Verification items for the finished model (mm, model axes). A direction names the side the tool comes from. Give positions to 0.01 mm unless a question says otherwise; leave off trailing zeros. Order: outer loops, then holes, each group sorted by start corner. A loop starts at its lowest first (then second) coordinate and runs counter-clockwise, first axis right, second up. Notation, with made-up numbers: (84, -37) - (121, -37) arc R11 ccw to (121, -22) - close; hole circle Ø8 at (65, -15.75). An arc over 180 degrees is marked (long way). Answer as a JSON object with one key per item and string values. Group by question number.
(1) Section check C-C (y = 82.5). Record the boundary of the cut face in (x, z).
(2) Depth check by flat-ended pin: pin 1 Ø16 at (x, z) = (3.5, 102) entering from -Y; pin 2 Ø8 at (x, z) = (-5, 85) entering from -Y; pin 3 Ø9.5 at (x, z) = (0, 99.82) entering from +Y; pin 4 Ø0.6 at (y, z) = (94, 93.5) entering from -X. Enter the tip coordinate at first touch or a pass-through.
(3) Section check D-D (y = -4.5). Record the boundary of the cut face in (x, z).
(4) Access from +Z, -Z, +X, -X, +Y, -Y to the whole of each face (thin tool, end or side, straight path). Record for faces 4 (the face through (19.077, 85.48, 85.907)), 5 (the face through (-2.7, 94.01, 94.62)).
(5) Section check B-B (z = 0). Record the boundary of the cut face in (x, y).
(6) Section check A-A (x = 0). Record the boundary of the cut face in (y, z), then the cut area to 3 significant figures.
(7) Mould release check, pull along Z, two halves, no side actions. Record for faces 1 (the face through (8.574, 93.986, 107.939)), 2 (the face through (47, 95, 76)), 3 (the face through (-28.441, 1.405, -8.956)): +Z half, -Z half, draft (parallel to the pull), parting line (faces both ways), or undercut.
(8) Thickness scan on line 1 (Z direction, x = 0, y = 94); line 2 (Z direction, x = 0, y = 80.5); line 3 (Z direction, x = 51, y = 75). Record the ranges inside material, lowest first.
```python
from build123d import *

# Parameters (mm, degrees)
VACIADO1_T              = -2
SALIENTE_EXTRUIR1_DEPTH = 2
CROQUIS3_R              = 5.855610057
CORTAR_EXTRUIR1_DEPTH   = 22
REDONDEO1_R             = 5


with BuildPart() as part:
    # Croquis1 → Revolución1 (revolve)
    with BuildSketch(Plane.XY, mode=Mode.PRIVATE) as revoluci_n1_sk:
        Polygon((0, 95), (0, -95), (10, -95), (19.509364421, -15), (90, 75), (90, 95), align=None)
    revolve(revoluci_n1_sk.sketch.rotate(Axis((0, 95, 0), (0, -1, 0)), 180), axis=Axis((0, 95, 0), (0, -1, 0)))

    # Vaciado1
    vaciado1_openings = [part.faces().sort_by_distance(p)[0] for p in [
        (0, -95, 0),
        (0, 95, 0),
    ]]
    offset(amount=VACIADO1_T, openings=vaciado1_openings, kind=Kind.INTERSECTION)

    # Croquis2 → Saliente-Extruir1 (add)
    with BuildSketch(Plane(origin=(0, 95, 0), x_dir=(1, 0, 0), z_dir=(0, 1, 0))):
        with BuildLine():
            Line((0, -109.4427191), (0, -90))
            ThreePointArc((0, -90), (-5.007758031, -89.860571774), (-10, -89.4427191))
            Line((-10, -89.4427191), (-10, -109.4427191))
            Line((-10, -109.4427191), (0, -109.4427191))
        make_face()
        with BuildLine():
            ThreePointArc((10, -89.4427191), (5.007758031, -89.860571774), (0, -90))
            Line((0, -90), (0, -109.4427191))
            Line((0, -109.4427191), (10, -109.4427191))
            Line((10, -109.4427191), (10, -89.4427191))
        make_face()
    extrude(amount=-SALIENTE_EXTRUIR1_DEPTH)

    # Croquis3 → Cortar-Extruir1 (cut)
    with BuildSketch(Plane(origin=(0, 95, 0), x_dir=(1, 0, 0), z_dir=(0, 1, 0))):
        with Locations(Location((0, -99.817771653, 0), (0, 0, 180))):
            Circle(CROQUIS3_R)
    extrude(amount=-CORTAR_EXTRUIR1_DEPTH, mode=Mode.SUBTRACT)

    # Redondeo1
    redondeo1_edges = [part.edges().sort_by_distance(p)[0] for p in [
        (10, 94, 109.4427191),
        (-10, 94, 109.4427191),
    ]]
    fillet(redondeo1_edges, radius=REDONDEO1_R)


solid = part.part
```
Solutions:
{
 "1": {"outline": "circle Ø180 at (0, 0); hole circle Ø176 at (0, 0)"},
 "2": {"pin 1": "stops at y = 93", "pin 2": "stops at y = 63.7", "pin 3": "passes through", "pin 4": "stops at x = -10"},
 "3": {"outline": "circle Ø55.47 at (0, 0); hole circle Ø50.39 at (0, 0)"},
 "4": {"face 4": "+Y", "face 5": "+Y, -Y"},
 "5": {"outline": "(-90, 75) - (-19.51, -15) - (-10, -95) - (-7.99, -95) - (-17.59, -14.21) - (-88, 75.69) - (-88, 95) - (-90, 95) - close; (7.99, -95) - (10, -95) - (19.51, -15) - (90, 75) - (90, 95) - (88, 95) - (88, 75.69) - (17.59, -14.21) - close"},
 "6": {"outline": "(-95, -10) - (-15, -19.51) - (75, -90) - (95, -90) - (95, -88) - (75.69, -88) - (-14.21, -17.59) - (-95, -7.99) - close; (-95, 7.99) - (-14.21, 17.59) - (75.69, 88) - (95, 88) - (95, 93.96) - (93, 93.96) - (93, 90) - (75, 90) - (-15, 19.51) - (-95, 10) - close; (93, 105.67) - (95, 105.67) - (95, 109.44) - (93, 109.44) - close", "area": "875 mm2"},
 "7": {"face 1": "+Z half", "face 2": "draft", "face 3": "undercut"},
 "8": {"line 1": "z = -90 to -88, 88 to 93.96, 105.67 to 109.44", "line 2": "z = -90 to -88, 88 to 90", "line 3": "z = -74.16 to -71.05, 71.05 to 74.16"}
}
